```python
from build123d import *

# Parameters (mm, degrees)
SKETCH_R  = 6.5
PAD_DEPTH = 8


with BuildPart() as part:
    # Sketch → Pad (new body)
    with BuildSketch(Plane.XY):
        with BuildLine():
            Line((-457, -40), (0, -40))
            Line((0, -40), (457, -40))
            ThreePointArc((457, -40), (459.12132, -39.12132), (460, -37))
            Line((460, -37), (460, -4))
            ThreePointArc((460, -4), (459.12132, -1.87868), (457, -1))
            Line((58, -1), (457, -1))
            Line((57, -1), (58, -1))
            Line((57, 50), (57, -1))
            Line((-57, 50), (57, 50))
            Line((-57, -1), (-57, 50))
            Line((-57, -1), (-58, -1))
            Line((-58, -1), (-457, -1))
            ThreePointArc((-457, -1), (-459.12132, -1.87868), (-460, -4))
            Line((-460, -37), (-460, -4))
            ThreePointArc((-460, -37), (-459.12132, -39.12132), (-457, -40))
        make_face()
        with Locations((-24, 12)):
            Circle(SKETCH_R, mode=Mode.SUBTRACT)
        with Locations((24, 12)):
            Circle(SKETCH_R, mode=Mode.SUBTRACT)
        with BuildLine():
            ThreePointArc((-453.5, -31), (-450, -34.5), (-446.5, -31))
            Line((-446.5, -31), (-446.5, -10))
            ThreePointArc((-446.5, -10), (-450, -6.5), (-453.5, -10))
            Line((-453.5, -31), (-453.5, -10))
        make_face(mode=Mode.SUBTRACT)
        with BuildLine():
            ThreePointArc((446.5, -31), (450, -34.5), (453.5, -31))
            Line((453.5, -31), (453.5, -10))
            ThreePointArc((453.5, -10), (450, -6.5), (446.5, -10))
            Line((446.5, -31), (446.5, -10))
        make_face(mode=Mode.SUBTRACT)
    extrude(amount=PAD_DEPTH)


solid = part.part
```
Could you check a few things on this model? Use its own coordinates, in mm. Give positions to 0.01 mm unless a question says otherwise; leave off trailing zeros. Write each loop counter-clockwise with the first axis right and the second up, starting at its lowest first coordinate (ties: lowest second). Pieces come first, ordered by that corner, then holes. Notation, with made-up numbers: (14.5, 61) -> (69.5, 61) arc R27 cw to (69.5, 77) -> close; hole circle Ø3 at (-7.75, 19.5). An arc over 180 degrees is marked (long way). Write each question's results on one line, items separated by ' | '.
1. I want a section at A-A, the plane z = 2.5. Write out the boundary of the cut face in (x, y), then the cut area to 3 significant figures.
Check sheet entries:
outline: (-460, -37) arc R3 ccw to (-457, -40) -> (457, -40) arc R3 ccw to (460, -37) -> (460, -4) arc R3 ccw to (457, -1) -> (57, -1) -> (57, 50) -> (-57, 50) -> (-57, -1) -> (-457, -1) arc R3 ccw to (-460, -4) -> close; hole (-453.5, -31) arc R3.5 ccw to (-446.5, -31) -> (-446.5, -10) arc R3.5 ccw to (-453.5, -10) -> close; hole circle Ø13 at (-24, 12); hole circle Ø13 at (24, 12); hole (446.5, -31) arc R3.5 ccw to (453.5, -31) -> (453.5, -10) arc R3.5 ccw to (446.5, -10) -> close | area: 41,000 mm²
2. I want a section at B-B, the plane x = 138.5. Write out the boundary of the cut face in (y, z), then the cut area to 3 significant figures.
Check sheet entries:
outline: (-40, 0) -> (-1, 0) -> (-1, 8) -> (-40, 8) -> close | area: 312 mm²
3. I want a section at C-C, the plane y = 30. Write out the boundary of the cut face in (x, z).
Check sheet entries:
outline: (-57, 0) -> (57, 0) -> (57, 8) -> (-57, 8) -> close
4. I need wall thicknesses on L1, parallel to X at y = -24, z = 3.75; L2, parallel to Y at x = 24, z = 5; L3, parallel to X at y = 17.5, z = 3. Which ranges of each line are inside material? Lowest first, please.
Check sheet entries:
L1: x = -460 to -453.5, -446.5 to 446.5, 453.5 to 460 | L2: y = -40 to 5.5, 18.5 to 50 | L3: x = -57 to -27.46, -20.54 to 20.54, 27.46 to 57
5. Will these pins go through, and if not, where does the flat tip stop? pin 1 Ø1.5 at (y, z) = (12.5, 2) entering from +X; pin 2 Ø4 at (y, z) = (17, 4.5) entering from -X; pin 3 Ø2.5 at (x, z) = (-283.5, 5) entering from +Y.
Check sheet entries:
pin 1: stops at x = 57 | pin 2: stops at x = -57 | pin 3: stops at y = -1
